```python
from build123d import *

# Parameters (mm, degrees)
F0_R     = 36.5125
F1_DEPTH = 180.975
F2_R     = 6.5484375
F3_DEPTH = 180.976
F4_R     = 9.525
F5_DEPTH = 14.2875
F6_R     = 12.7635
F7_DEPTH = 25.4
F8_SIZE  = 1.5875
F9_SIZE2 = 19.05
F9_SIZE  = 4.7625


with BuildPart() as f1:
    # F0 (on Right) → F1 (new body)
    with BuildSketch(Plane.YZ):
        Circle(F0_R)
    extrude(amount=-F1_DEPTH)

    # F2 (on face) → F3 (cut, through all)
    with BuildSketch(Plane.YZ):
        Circle(F2_R)
    extrude(amount=-F3_DEPTH, mode=Mode.SUBTRACT)

    # F4 (on face) → F5 (cut)
    with BuildSketch(Plane.YZ):
        Circle(F4_R)
    extrude(amount=-F5_DEPTH, mode=Mode.SUBTRACT)

    # F6 (on face) → F7 (cut)
    with BuildSketch(Plane(origin=(-180.975, 0, 0), x_dir=(0, -1, 0), z_dir=(-1, 0, 0))):
        Circle(F6_R)
    extrude(amount=-F7_DEPTH, mode=Mode.SUBTRACT)

    # F8
    f8_edges = [f1.edges().sort_by_distance(p)[0] for p in [
        (0, -9.525, 0),
        (-180.975, -36.5125, 0),
        (-180.975, 12.7635, 0),
    ]]
    chamfer(f8_edges, length=F8_SIZE)

    # F9
    f9_edges = [f1.edges().sort_by_distance(p)[0] for p in [
        (0, -36.5125, 0),
    ]]
    f9_side = f1.faces().sort_by_distance((0, -12.145229, 0))[0]
    chamfer(f9_edges, length=F9_SIZE, length2=F9_SIZE2, reference=f9_side)


solid = f1.part
```
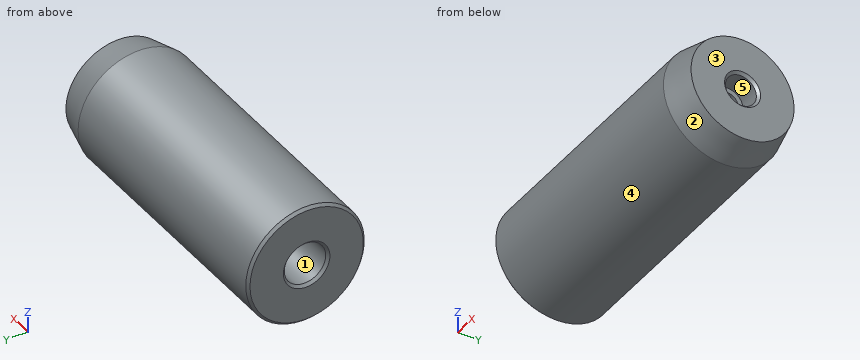
The model under review builds one solid part; all positions refer to its coordinate system, in mm. Face numbers are marked on the shaded views. A direction names the side the tool comes from. Round coordinates to 2 decimals unless told otherwise and drop trailing zeros. Order: outer loops, then holes, each group sorted by start corner. A loop starts at its lowest first (then second) coordinate and runs counter-clockwise, first axis right, second up. Notation, with made-up numbers: (-30, -27.5) -> (-14, -27.5) arc R22 ccw to (-14, -0.5) -> close; hole circle Ø3 at (47, 18.5). An arc over 180 degrees is marked (long way). One line per item, written item: value. Start each with the question number.
Q1. Wall thickness on line 1 (Z direction, x = -165.25, y = 0); line 2 (Z direction, x = -9, y = 0) (3 decimals); line 3 (Y direction, x = -126, z = -3): over which ranges is each line inside the solid? List them lowest first.
Q2. Take a section at C-C (x = -42). Write out the cut boundary in (y, z) (1 decimal).
Q3. Machinability: for the marked faces 1 and 2, which of the approach directions +Z, -Z, +X, -X, +Y, -Y give a long, thin tool a straight path to every point of the face, cutting with its end or side? Answer none if there is none.
Q4. Mouldability with a two-part tool opening along Y and no side actions: class the marked faces 3, 4 and 5 as released by +Y, released by -Y, zero draft, split by the parting line, or undercut.
Q5. Clearance check with flat-ended pins moving along their axes: pin 1 Ø1 at (x, y) = (-106.5, 23) entering from -Z; pin 2 Ø6 at (x, y) = (-31, -23) entering from -Z; pin 3 Ø21 at (y, z) = (0, 0) entering from +X. State where each tip first meets the part, or that it passes through.
Reported:
1. line 1: z = -36.51 to -12.76, 12.76 to 36.51
1. line 2: z = -34 to -9.525, 9.525 to 34
1. line 3: y = -36.39 to -5.82, 5.82 to 36.39
2. outline: circle Ø73 at (0, 0); hole circle Ø13.1 at (0, 0)
3. face 1: -X
3. face 2: +X
4. face 3: zero draft
4. face 4: split by the parting line
4. face 5: undercut
5. pin 1: stops at z = -28.76
5. pin 2: stops at z = -30.55
5. pin 3: stops at x = -0.61
